Design review of the part built by this model. Coordinates are the model's own, in mm. A direction names the side the tool comes from. Coordinates: 2 decimals unless noted, no trailing zeros. Loops run counter-clockwise (first coordinate to the right, second up) from the corner with the lowest first, then second, coordinate; pieces in that order, holes last. Notation, with made-up numbers: (29, 25) -> (49, 25) arc R23 cw to (49, 37) -> close; hole circle Ø4 at (-13, 51.5). An arc over 180 degrees is marked (long way). One line per item, written item: value. Start each with the question number.
1. For probe 1 along X at (y, z) = (-41.25, 5); probe 2 along X at (y, z) = (-20, 1.5); probe 3 along Y at (x, z) = (14.5, 8.75), list the stretches that pass through material, from the lowest coordinate up.
2. Add section C-C on z = 9.25. Write out the cut boundary in (x, y).
3. Machinability: for faces 1 (the cylindrical face through (1.73, -41.61, 5.86)), 2 (the flat face through (14, -47.191, 5)), which of the approach directions +Z, -Z, +X, -X, +Y, -Y give a long, thin tool a straight path to every point of the face, cutting with its end or side? Answer none if there is none.
4. Add section A-A on y = -27. Write out the cut boundary in (x, z).
5. Draft analysis for pull direction X (two halves, no side actions). For faces 3 (the conical face through (3.973, -34.764, 5.022)), 4 (the cylindrical face through (34.406, -16.943, 5.055)), 5 (the flat face through (35.472, -27, 5)), state which applies: pulls with the +X half, pulls with the -X half, needs draft (parallel to the pull), parting line crosses it, or undercut.
6. Add section B-B on x = 8.5. Write out the cut boundary in (y, z).
7. Insertion check: pin 1 (1 mm diameter, centred on x = 2, y = -10.5, fed in from -Z); pin 2 (4.5 mm diameter, centred on x = 4.47, z = 5, fed in from -Y). Each pin has a flat end and moves straight along its axis. Give the tip position at first contact, or say it passes through.
```python
from build123d import *

# Parameters (mm, degrees)
F1_DEPTH = 10
F3_D     = 22
F4_D     = 8
F6_D     = 2.5
F6_DEPTH = 5
F6_TIP   = 0.7510757738
F8_D     = 5.75
F8_DEPTH = 11
F8_TIP   = 1.7274742797


# Not quite as in the source:
# - a feature names something its author has since deleted; it is built from what else it names


with BuildPart() as f1:
    # F0 (on Top) → F1 (new body)
    with BuildSketch(Plane.XY):
        Polygon((-6.5280715935, -6.1914156973), (-6.5280715935, -47.1914156973), (35.4719284065, -47.1914156973), (35.4719284065, -6.1914156973), (31.4719284065, -2.1914156973), (-2.5280715935, -2.1914156973), align=None)
    extrude(amount=F1_DEPTH)

    # F3 (through all)
    with Locations(Plane.XY.offset(10)):
        with Locations((7.4719284065, -19.1914156973)):
            Hole(F3_D / 2)

    # F4 (through all)
    with Locations(Plane.XY.offset(10)):
        with Locations((29.4719284065, -19.1914156973)):
            Hole(F4_D / 2)

    # F6
    with Locations(Plane.YZ.offset(35.4719284065)):
        with Locations((-18.1914156973, 5)):
            Hole(F6_D / 2, depth=F6_DEPTH)
            with Locations((0, 0, -(F6_DEPTH + F6_TIP / 2))):  # 118° drill point
                Cone(0, F6_D / 2, F6_TIP, mode=Mode.SUBTRACT)

    # F8
    with Locations(Plane.XZ.offset(47.1914156973)):
        with Locations((28.4719284065, 5), (4.4719284065, 5)):
            Hole(F8_D / 2, depth=F8_DEPTH)
            with Locations((0, 0, -(F8_DEPTH + F8_TIP / 2))):  # 118° drill point
                Cone(0, F8_D / 2, F8_TIP, mode=Mode.SUBTRACT)


solid = f1.part
```
Worked answers:
1. probe 1: x = -6.53 to 1.6, 7.35 to 25.6, 31.35 to 35.47
1. probe 2: x = -6.53 to -3.5, 18.44 to 25.55, 33.39 to 35.47
1. probe 3: y = -47.19 to -27.65, -10.73 to -2.19
2. outline: (-6.53, -47.19) -> (35.47, -47.19) -> (35.47, -6.19) -> (31.47, -2.19) -> (-2.53, -2.19) -> (-6.53, -6.19) -> close; hole circle Ø22 at (7.47, -19.19); hole circle Ø8 at (29.47, -19.19)
3. face 1: -Y
3. face 2: +Z, -Z, +X, -X, -Y
4. outline: (-6.53, 0) -> (-0.28, 0) -> (-0.28, 10) -> (-6.53, 10) -> close; (15.22, 0) -> (35.47, 0) -> (35.47, 10) -> (15.22, 10) -> close
5. face 3: undercut
5. face 4: needs draft
5. face 5: pulls with the +X half
6. outline: (-47.19, 0) -> (-30.14, 0) -> (-30.14, 10) -> (-47.19, 10) -> close; (-8.24, 0) -> (-2.19, 0) -> (-2.19, 10) -> (-8.24, 10) -> close
7. pin 1: passes through
7. pin 2: stops at y = -35.82
